from build123d import *

# Parameters (mm, degrees)
SKETCH_1_W      = 150
SKETCH_1_H      = 150
EXTRUDE_1_DEPTH = 110
SHELL_1_T       = -2
EXTRUDE_START   = -60
EXTRUDE_2_DEPTH = 2
FILLET_1_R      = 10


with BuildPart() as part:
    # 草图1 → 凸台-拉伸1 (new body)
    with BuildSketch(Plane.XY):
        Rectangle(SKETCH_1_W, SKETCH_1_H)
    extrude(amount=EXTRUDE_1_DEPTH)

    # 抽壳1
    shell_1_openings = [part.faces().sort_by_distance(p)[0] for p in [
        (0, 0, 110),
    ]]
    offset(amount=SHELL_1_T, openings=shell_1_openings, kind=Kind.INTERSECTION)

    # 草图2 → 凸台-拉伸2 (add)
    with BuildSketch(Plane.XY.offset(110).offset(EXTRUDE_START)):
        with BuildLine():
            Line((-19.944653056, -75), (-17.301604129, -78.907070498))
            ThreePointArc((-17.301604129, -78.907070498), (-13.28346315, -82.348966768), (-8.071553148, -83.258967309))
            Line((-8.071553148, -83.258967309), (0, -82.490938419))
            Line((0, -82.490938419), (8.071553148, -83.258967309))
            ThreePointArc((8.071553148, -83.258967309), (13.28346315, -82.348966768), (17.301604129, -78.907070498))
            Line((17.301604129, -78.907070498), (19.944653056, -75))
            Line((19.944653056, -75), (14.314326214, -75))
            Line((14.314326214, -75), (14.932632038, -70.214502915))
            ThreePointArc((14.932632038, -70.214502915), (11.617573252, -76.443569186), (5.01506981, -78.933113254))
            Line((5.01506981, -78.933113254), (-5.01506981, -78.933113254))
            ThreePointArc((-5.01506981, -78.933113254), (-11.617573252, -76.443569186), (-14.932632038, -70.214502915))
            Line((-14.932632038, -70.214502915), (-14.314326214, -75))
            Line((-14.314326214, -75), (-19.944653056, -75))
        make_face()
    extrude(amount=EXTRUDE_2_DEPTH)

    # 圆角1
    # the kernel refuses this fillet: 10 mm, written as the material it adds along each edge
    with BuildSketch(Plane(origin=(19.944653056, -75, 50), x_dir=(1, 0, 0), z_dir=(0, 0, 1))) as fillet_1_piece_1:
        with BuildLine():
            CenterArc((5.297648539, -10), FILLET_1_R, 90, 54.21089853)
            Line((-2.814102182, -4.151966123), (-3.625277254, -3.567162735))
            ThreePointArc((-3.625277254, -3.567162735), (-3.471329325, -3.346756673), (-0.828280398, 0.560313825))
            Line((-0.828280398, 0.560313825), (0, 1))
            Line((0, 1), (5.297648539, 1))
            Line((5.297648539, 1), (5.297648539, 0))
        make_face()
    extrude(amount=2)
    with BuildSketch(Plane(origin=(-19.944653056, -75, 50), x_dir=(-1, 0, 0), z_dir=(0, 0, 1))) as fillet_1_piece_2:
        with BuildLine():
            CenterArc((5.297648539, 10), FILLET_1_R, 215.78910147, 54.21089853)
            Line((-2.814102182, 4.151966123), (-3.625277254, 3.567162735))
            ThreePointArc((-3.625277254, 3.567162735), (-3.471329325, 3.346756673), (-0.828280398, -0.560313825))
            Line((-0.828280398, -0.560313825), (0, -1))
            Line((0, -1), (5.297648539, -1))
            Line((5.297648539, -1), (5.297648539, 0))
        make_face()
    extrude(amount=2)


solid = part.part
Could you check a few things on this model? Use its own coordinates, in mm. A direction names the side the tool comes from. Give positions to 0.01 mm unless a question says otherwise; leave off trailing zeros. Write each loop counter-clockwise with the first axis right and the second up, starting at its lowest first coordinate (ties: lowest second). Pieces come first, ordered by that corner, then holes. Notation, with made-up numbers: (15.5, 7.25) -> (70.5, 7.25) arc R26 ccw to (70.5, 44.25) -> close; hole circle Ø7 at (62, -35). An arc over 180 degrees is marked (long way). Answer as a JSON object with one key per item and string values.
Q1. Which directions (+Z, -Z, +X, -X, +Y, -Y) give clear straight access to the entire face, cutting with the end or side of a thin tool? Please do faces 1 (the flat face through (0, -80, 52)), 2 (the flat face through (-73, -1, 55)), 3 (the flat face through (0, -80, 50)).
Taken from the geometry:
{"face 1": "+Z, +X, -X, -Y", "face 2": "+Z", "face 3": "-Z, +X, -X, -Y"}
Q2. Will these pins go through, and if not, where does the flat tip stop? pin 1 Ø8 at (x, y) = (18, 23) entering from +Z; pin 2 Ø0.9 at (x, y) = (-14.5, -71.5) entering from +Z; pin 3 Ø4 at (x, y) = (-10.5, -79) entering from -Z.
Taken from the geometry:
{"pin 1": "stops at z = 2", "pin 2": "stops at z = 52", "pin 3": "stops at z = 50"}
Q3. Suppose I cut it at A-A on z = 88. Write out the boundary of the cut face in (x, y).
Taken from the geometry:
{"outline": "(-75, -75) -> (75, -75) -> (75, 75) -> (-75, 75) -> close; hole (-73, -73) -> (73, -73) -> (73, 73) -> (-73, 73) -> close"}
Q4. We'd pull the mould along Y, two halves only. Please class faces 4 (the flat face through (-1, -73, 55)), 5 (the flat face through (-1, 1, 0)), 6 (the flat face through (-1, 75, 54)), 7 (the flat face through (73, -1, 55)): released by +Y, released by -Y, zero draft, split by the parting line, or undercut.
Taken from the geometry:
{"face 4": "undercut", "face 5": "zero draft", "face 6": "released by +Y", "face 7": "undercut"}
Q5. Please list where these lines run through material, in increasing order: L1, parallel to X at y = 48.5, z = 89; L2, parallel to Z at x = 15.5, y = 9.
Taken from the geometry:
{"L1": "x = -75 to -73, 73 to 75", "L2": "z = 0 to 2"}
Q6. Suppose I cut it at B-B on y = -54.5. Write out the boundary of the cut face in (x, z), then the cut area to 3 significant figures.
Taken from the geometry:
{"outline": "(-75, 0) -> (75, 0) -> (75, 110) -> (73, 110) -> (73, 2) -> (-73, 2) -> (-73, 110) -> (-75, 110) -> close", "area": "732 mm²"}
